Autodesk Inventor part; units mm, degrees
ref_plane "YZ Plane" through (0, 0, 0) normal (1, 0, 0) x (0, 1, 0)
ref_plane "XZ Plane" through (0, 0, 0) normal (0, 1, 0) x (-1, 0, 0)
ref_plane "XY Plane" through (0, 0, 0) normal (0, 0, 1) x (1, 0, 0)
sketch "Boceto1" plane through (0, 0, 0) normal (0, 0, 1) x (1, 0, 0)
  circle A0 centre (0, 0) radius 57.15
  circle A1 centre (101.6, 0) radius 44.45
  circle A2 centre (-31.75, 47.519) radius 11.1125
  circle A3 centre (-31.75, -47.519) radius 11.1125
  circle A4 centre (114.3, 42.5971) radius 11.1125
  circle A5 centre (114.3, -42.5971) radius 11.1125
  line L0 (7.1437, 56.7018) -> (107.1562, 44.1014)
  circle A6 centre (44.45, 52.0016) radius 11.1125
  line L1 (7.1437, -56.7018) -> (107.1562, -44.1014)
  circle A7 centre (44.45, -52.0016) radius 11.1125
  dimension "d0" = 114.3
  dimension "d1" = 88.9
  dimension "d2" = 203.2
  dimension "d3" = 22.225
  dimension "d4" = 22.225
  dimension "d7" = 22.225
  dimension "d8" = 22.225
  dimension "d11" = 22.225
  dimension "d13" = 0
  dimension "d14" = 22.225
  dimension "d27" = 12.7
  dimension "d28" = 12.7
  dimension "d29" = 44.45
  dimension "d30" = 44.45
  dimension "d31" = 31.75
  dimension "d32" = 31.75
extrude "Extrusión1" add sketch "Boceto1" along normal blind 4.445
sketch "Boceto2" plane through (0, 0, 4.445) normal (0, 0, 1) x (1, 0, 0)
  arc A0 (-21.9537, 52.7651) -> (-40.3458, 40.4764) centre (-31.75, 47.519) ccw
  circle A1 centre (-31.75, 47.519) radius 4.7625
  arc A2 (-40.3458, -40.4764) -> (-21.9537, -52.7651) centre (-31.75, -47.519) ccw
  circle A3 centre (-31.75, -47.519) radius 4.7625
  arc A4 (33.4247, -53.3907) -> (55.4753, -50.6125) centre (44.45, -52.0016) ccw
  circle A5 centre (44.45, -52.0016) radius 4.7625
  arc A6 (55.4753, 50.6125) -> (33.4247, 53.3907) centre (44.45, 52.0016) ccw
  circle A7 centre (44.45, 52.0016) radius 4.7625
  arc A8 (124.4689, 38.1158) -> (103.3657, 44.5789) centre (114.3, 42.5971) ccw
  circle A9 centre (114.3, 42.5971) radius 4.7625
  arc A10 (103.3657, -44.5789) -> (124.4689, -38.1158) centre (114.3, -42.5971) ccw
  circle A11 centre (114.3, -42.5971) radius 4.7625
  point P0 (0, 0)
  dimension "d18" = 9.525
  dimension "d19" = 9.525
  dimension "d20" = 9.525
  dimension "d21" = 9.525
  dimension "d22" = 9.525
  dimension "d23" = 9.525
extrude "Extrusión2" cut sketch "Boceto2" against normal up to surface (4.445 mm away)
fillet "Empalme1" radius 6.35 12 edges at (-21.9537, -52.7651, 2.2225) (-40.3458, -40.4764, 2.2225) (33.4247, -53.3907, 2.2225) (55.4753, -50.6125, 2.2225) (124.4689, -38.1158, 2.2225) (-40.3458, 40.4764, 2.2225) (-21.9537, 52.7651, 2.2225) (33.4247, 53.3907, 2.2225) (55.4753, 50.6125, 2.2225) (103.3657, 44.5789, 2.2225) (124.4689, 38.1158, 2.2225) (103.3657, -44.5789, 2.2225)
sketch "Boceto3" plane through (0, 0, 0) normal (0, 0, -1) x (-1, 0, 0)
  circle A0 centre (0, 0) radius 7.1437
  circle A1 centre (0, -45) radius 6.35
  circle A2 centre (0, 45) radius 6.35
  line L0 (0, -45) -> (0, 0)
  line L1 (0, 0) -> (0, 45)
  dimension "d33" = 14.2875
  dimension "d34" = 12.7
  dimension "d35" = 12.7
  dimension "d36" = 45
  dimension "d37" = 45
extrude "Extrusión3" cut sketch "Boceto3" against normal up to surface (4.445 mm away)
sketch "Boceto4" plane through (0, 0, 4.445) normal (0, 0, 1) x (1, 0, 0)
  circle A0 centre (93.4212, 0) radius 5.5563
  line L0 (65.4212, -28) -> (121.4212, -28)
  line L1 (121.4212, -28) -> (121.4212, 28)
  line L2 (121.4212, 28) -> (65.4212, 28)
  line L3 (65.4212, 28) -> (65.4212, -28)
  line L4 (69.6712, -23.75) -> (117.1712, -23.75)
  line L5 (117.1712, -23.75) -> (117.1712, 23.75)
  line L6 (117.1712, 23.75) -> (69.6712, 23.75)
  line L7 (69.6712, 23.75) -> (69.6712, -23.75)
  circle A1 centre (74.8306, -23.75) radius 2.7781
  circle A2 centre (112.0118, -23.75) radius 2.7781
  circle A3 centre (122.3306, -23.75) radius 2.7781
  circle A4 centre (64.5118, -23.75) radius 2.7781
  line L8 (64.5118, -26.5281) -> (74.8306, -26.5281)
  line L9 (64.5118, -20.9719) -> (74.8306, -20.9719)
  line L10 (112.0118, -26.5281) -> (122.3306, -26.5281)
  line L11 (122.3306, -20.9719) -> (112.0118, -20.9719)
  circle A5 centre (74.8306, 23.75) radius 2.7781
  circle A6 centre (64.5118, 23.75) radius 2.7781
  line L12 (64.5118, 20.9719) -> (74.8306, 20.9719)
  line L13 (64.5118, 26.5281) -> (74.8306, 26.5281)
  circle A7 centre (112.0118, 23.75) radius 2.7781
  circle A8 centre (122.3306, 23.75) radius 2.7781
  line L14 (112.0118, 20.9719) -> (122.3306, 20.9719)
  line L15 (112.0118, 26.5281) -> (122.3306, 26.5281)
  circle A9 centre (98.5806, 0) radius 5.5563
  circle A10 centre (88.2618, 0) radius 5.5563
  line L16 (98.5806, 5.5563) -> (88.2618, 5.5563)
  line L17 (98.5806, -5.5563) -> (88.2618, -5.5563)
  point P0 (0, 0)
  dimension "d40" = 11.1125
  dimension "d41" = 56
  dimension "d42" = 56
  dimension "d43" = 28
  dimension "d44" = 28
  dimension "d45" = 0
  dimension "d46" = 93.4212
  dimension "d47" = 47.5
  dimension "d48" = 47.5
  dimension "d49" = 23.75
  dimension "d50" = 23.75
  dimension "d57" = 5.5563
  dimension "d58" = 5.1594
  dimension "d59" = 5.5563
  dimension "d60" = 5.5563
  dimension "d61" = 5.1594
  dimension "d62" = 5.1594
  dimension "d63" = 5.5563
  dimension "d64" = 5.1594
  dimension "d65" = 0
  dimension "d66" = 5.5563
  dimension "d67" = 5.5563
  dimension "d68" = 5.1594
  dimension "d69" = 5.1594
  dimension "d70" = 0
  dimension "d71" = 5.5563
  dimension "d72" = 5.5563
  dimension "d73" = 5.1594
  dimension "d74" = 5.1594
  dimension "d75" = 0
  dimension "d78" = 11.1125
  dimension "d79" = 11.1125
  dimension "d80" = 5.1594
  dimension "d81" = 5.1594
extrude "Extrusión4" cut sketch "Boceto4" against normal up to next contours A0 A9 A10 | A0 A9 | A9 A10 A0 | A0 L16 A9 | A9 L17 A0 | A0 A10 A9 | A0 A10 L16 | A10 A9 | A9 A10 A0 | L17 A10 A0 | A0 A10 | L8 A4 L3 | L3 A4 L9 L7 L4 A1 L8 | L10 A2 L4 L5 L11 L1 A3 | L1 A3 L10 | A4 L3 | L3 A4 | A1 L4 | A3 L1 | L1 A3 | A2 L4 | A4 L9 L3 | L4 A1 | L4 L7 L9 A1 | L1 L11 A3 | A2 L11 L5 L4 | L4 A2 | L12 A6 L3 | L3 A6 L13 A5 L6 L7 L12 | L14 L5 L6 A7 L15 L1 A8 | L1 A8 L14 | A6 L3 | L3 A6 | L7 L6 A5 L12 | A8 L1 | L1 A8 | L14 A7 L6 L5 | A6 L13 L3 | A5 L6 | L1 L15 A8 | A7 L6 | A5 L6 | L6 A7
sketch "Boceto5" plane through (0, 0, 4.445) normal (0, 0, 1) x (1, 0, 0)
  line L0 (50.8, -13.7453) -> (-50.8, -13.7453)
  line L1 (-50.8, -13.7453) -> (-50.8, -114.3)
  line L2 (-50.8, -114.3) -> (50.8, -114.3)
  line L3 (50.8, -114.3) -> (50.8, -13.7453)
  arc A0 (7.1437, 56.7018) -> (-17.8783, 54.2816) centre (0, 0) ccw
  arc A1 (7.1437, 56.7018) -> (-17.8783, 54.2816) centre (0, 0) ccw
  line L4 (0, 57.15) -> (7.6634, 57.15)
  arc A2 (127.9228, -35.8178) -> (127.9228, 35.8178) centre (101.6, 0) ccw
  line L5 (146.05, 0) -> (146.05, -27.5116)
  dimension "d82" = 101.6
  dimension "d84" = 171.45
  dimension "d85" = 95.25
extrude "Extrusión5" add sketch "Boceto5" against normal up to surface (4.445 mm away)
extrude "Extrusión6" cut sketch "Boceto2" against normal up to next contours A3 | A5
sketch "Boceto7" plane through (0, 0, 4.445) normal (0, 0, 1) x (1, 0, 0)
  circle A0 centre (31.75, -69.85) radius 4.3656
  circle A1 centre (31.75, -76.2) radius 4.3656
  line L0 (50.8, -114.3) -> (50.8, -61.1211)
  line L1 (-50.8, -114.3) -> (50.8, -114.3)
  line L2 (36.1156, -69.85) -> (36.1156, -76.2)
  line L3 (27.3844, -69.85) -> (27.3844, -76.2)
  circle A2 centre (31.75, -95.25) radius 4.3656
  circle A3 centre (31.75, -101.6) radius 4.3656
  line L4 (36.1156, -95.25) -> (36.1156, -101.6)
  line L5 (27.3844, -101.6) -> (27.3844, -95.25)
  point P0 (0, 0)
  dimension "d90" = 8.7312
  dimension "d91" = 8.7312
  dimension "d92" = 19.05
  dimension "d93" = 44.45
  dimension "d94" = 38.1
  dimension "d95" = 0
  dimension "d96" = 8.7312
  dimension "d97" = 8.7312
  dimension "d98" = 19.05
  dimension "d99" = 19.05
  dimension "d100" = 12.7
  dimension "d101" = 0
extrude "Extrusión7" cut sketch "Boceto7" against normal up to next
mirror "Simetría1" about plane through (0, 0, 0) normal (1, 0, 0) of "Extrusión7"
fillet "Empalme2" radius 6.35 4 edges at (-50.8, -26.1817, 2.2225) (-50.8, -114.3, 2.2225) (50.8, -61.1211, 2.2225) (50.8, -114.3, 2.2225)
extrude "Extrusión8" cut sketch "Boceto3" against normal up to next contours A1
equation "\"d16\" = t"
equation "\"d18\" = Q"
equation "\"d19\" = Q"
equation "\"d20\" = Q"
equation "\"d21\" = Q"
equation "\"d22\" = Q"
equation "\"d23\" = Q"
equation "\"d33\" = DF"
equation "\"d34\" = NF"
equation "\"d35\" = NF"
equation "\"d40\" = DM"
equation "\"d41\" = AM"
equation "\"d42\" = AM"
equation "\"d43\" = 0.5 * AM"
equation "\"d44\" = 0.5 * AM"
equation "\"d47\" = BM"
equation "\"d48\" = BM"
equation "\"d49\" = 0.5 * BM"
equation "\"d50\" = 0.5 * BM"
equation "\"d57\" = NM"
equation "\"d59\" = NM"
equation "\"d60\" = NM"
equation "\"d63\" = NM"
equation "\"d66\" = NM"
equation "\"d67\" = NM"
equation "\"d71\" = NM"
equation "\"d72\" = NM"
equation "\"d78\" = DM"
equation "\"d79\" = DM"
equation "\"d90\" = DH"
equation "\"d91\" = DH"
equation "\"d96\" = DH"
equation "\"d97\" = DH"
equation "\"t\" = 4.445"
equation "\"Q\" = 9.525"
equation "\"DF\" = 14.2875"
equation "\"NF\" = 12.7"
equation "\"DM\" = 11.1125"
equation "\"NM\" = 5.55625"
equation "\"CM\" = 93.4212"
equation "\"AM\" = 56"
equation "\"BM\" = 47.5"
equation "\"DH\" = 8.73125"
properties part number "CAR REDUCTION PLATE II"
CAD build for the part. Positions are in the model's coordinates, mm. A direction names the side the tool comes from. Round coordinates to 2 decimals unless told otherwise and drop trailing zeros. Loops run counter-clockwise (first coordinate to the right, second up) from the corner with the lowest first, then second, coordinate; pieces in that order, holes last. Notation, with made-up numbers: M 40,57.25 L 44,57.25 A10 ccw 44,62.25 Z; hole C -17.5,15.25 d6. An arc over 180 degrees is marked long. Use a Markdown table: item, result. Add a question column.
(1) Drill centre lines: line 1 (Y direction, x = 0, z = 1.8); line 2 (X direction, y = -102, z = 4.1); line 3 (Y direction, x = -31.75, z = 2.55). Where is each one in solid material? Low to high.
(2) Cut at D-D (z = 1.25). State how many separate pieces and enclosed holes the cut face has, and give its area (3 significant figures).
(3) Which spindle directions (+Z, -Z, +X, -X, +Y, -Y) get a long thin tool onto all of the face, cutting with end or side? Do faces 1 (the face through (70, -20.972, 2)), 2 (the face through (45.65, 63.05, 2.19)). Say none if no direction does.
(4) Cut at C-C (x = 31.75). Give the cut face in (y, z) (3 decimals), and give its area (3 significant figures).
(5) Cut at A-A (y = -98). Give the cut face in (x, z) (3 decimals), and give its area (3 significant figures).
(6) Pull direction Y, two halves, no side cores. Call faces 3 (the face through (54.212, -57.311, 2.191)), 4 (the face through (50.8, -86, 2)), 5 (the face through (-56.727, 6.944, 2.191)), 6 (the face through (125.11, -23.81, 2.25)): +Y half, -Y half, draft (parallel to the pull), parting line (faces both ways), or undercut.
(7) Flat gauge pins, fed straight in: pin 1 (7.5 mm diameter, centred on x = 44.45, y = 52, fed in from +Z); pin 2 (1.3 mm diameter, centred on x = 116.5, z = 2.5, fed in from +Y); pin 3 (1 mm diameter, centred on y = -89, z = 4, fed in from -X); pin 4 (2 mm diameter, centred on x = -32.5, z = 2.5, fed in from +Y). Where does each tip first touch, or does it go through?
(8) Cut at B-B (x = 0). Give the cut face in (y, z) (3 decimals), and give its area (3 significant figures).
Geometry says:
| question | item | result |
|---|---|---|
| 1 | line 1 | y = -114.3 to -51.35, -38.65 to -7.14, 7.14 to 38.65, 51.35 to 57.15 |
| 1 | line 2 | x = -50.8 to -36.1, -27.4 to 27.4, 36.1 to 50.8 |
| 1 | line 3 | y = -114.3 to -105.97, -90.88 to -80.57, -65.48 to -52.28, -42.76 to 42.76, 52.28 to 58.63 |
| 2 | separate pieces | 1 |
| 2 | enclosed holes | 18 |
| 2 | area | 24,100 mm² |
| 3 | face 1 | +Z, -Z |
| 3 | face 2 | +Z, -Z, +Y |
| 4 | outline | M -114.3,0 L -105.966,0 L -105.966,4.445 L -114.3,4.445 Z; M -90.884,0 L -80.566,0 L -80.566,4.445 L -90.884,4.445 Z; M -65.484,0 L 54.563,0 L 54.563,4.445 L -65.484,4.445 Z |
| 4 | area | 617 mm² |
| 5 | outline | M -50.8,0 L -36.116,0 L -36.116,4.445 L -50.8,4.445 Z; M -27.384,0 L 27.384,0 L 27.384,4.445 L -27.384,4.445 Z; M 36.116,0 L 50.8,0 L 50.8,4.445 L 36.116,4.445 Z |
| 5 | area | 374 mm² |
| 6 | face 3 | -Y half |
| 6 | face 4 | draft |
| 6 | face 5 | parting line |
| 6 | face 6 | undercut |
| 7 | pin 1 | passes through |
| 7 | pin 2 | stops at y = 53.6 |
| 7 | pin 3 | stops at x = -50.8 |
| 7 | pin 4 | stops at y = 58.63 |
| 8 | outline | M -114.3,0 L -51.35,0 L -51.35,4.445 L -114.3,4.445 Z; M -38.65,0 L -7.144,0 L -7.144,4.445 L -38.65,4.445 Z; M 7.144,0 L 38.65,0 L 38.65,4.445 L 7.144,4.445 Z; M 51.35,0 L 57.15,0 L 57.15,4.445 L 51.35,4.445 Z |
| 8 | area | 586 mm² |
